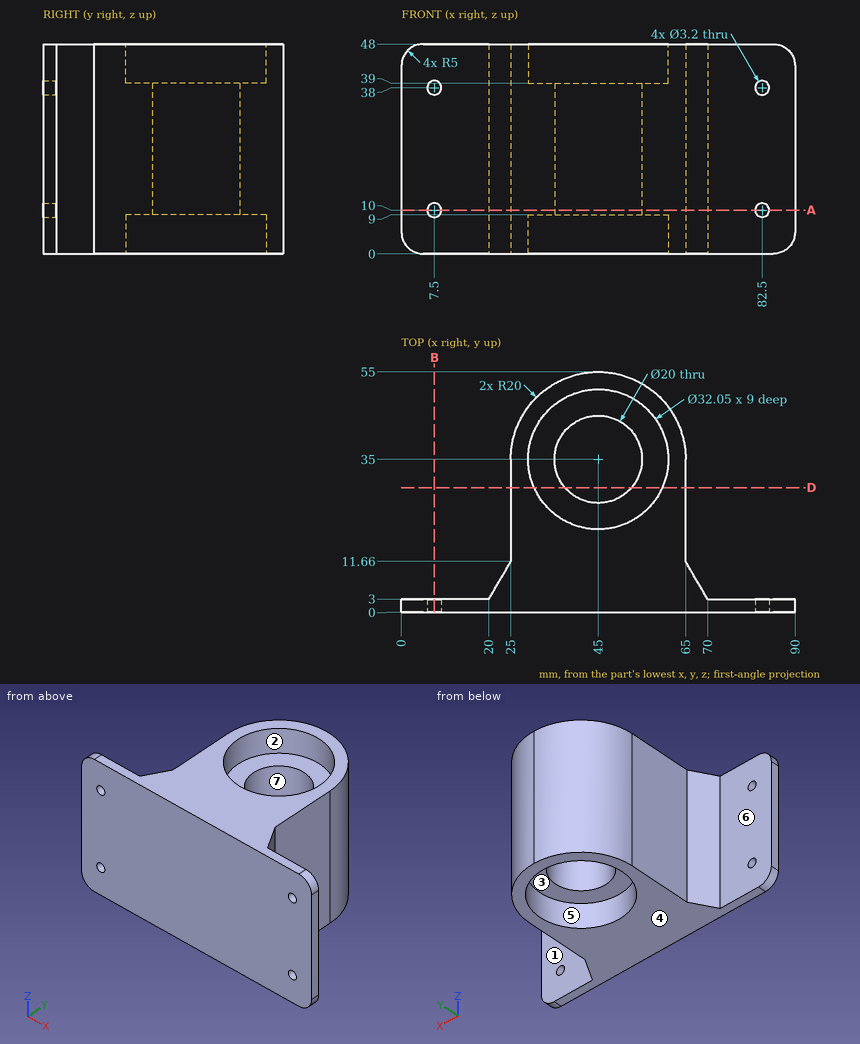
For this review, use the dimensioned drawing (mm, ordinates from the lowest corner) and the shaded views. A direction names the side the tool comes from. Give positions to 0.01 mm unless a question says otherwise; leave off trailing zeros. Write each loop counter-clockwise with the first axis right and the second up, starting at its lowest first coordinate (ties: lowest second). Pieces come first, ordered by that corner, then holes. Notation, with made-up numbers: M 55,27 L 69,27 A22 cw 69,48 Z; hole C -25,6.5 d10. An arc over 180 degrees is marked long. Answer as a JSON object with one key per item and string values. Group by question number.
Item 1: Consider section A-A on z = 10. Count the separate pieces of the cut face and the enclosed holes in it, plus the area to 3 significant figures.
Item 2: Consider section D-D on y = 28.5. Write out the cut boundary in (x, z), plus the area to 3 significant figures.
Item 3: Tool access review of the marked faces 1, 2 and 3: name each direction out of +Z, -Z, +X, -X, +Y, -Y from which nothing blocks a thin tool from reaching the whole face with its end or side.
Item 4: For probe 1 along X at (y, z) = (2.3, 38); probe 2 along Z at (x, y) = (82.5, 1.7); probe 3 along Y at (x, z) = (45, 24), list the stretches that pass through material, from the lowest coordinate up. Write a range as [from, to].
Item 5: For pin 1 Ø10 at (y, z) = (24, 21.5) entering from -X; pin 2 Ø1.9 at (x, z) = (7.5, 38) entering from +Y; pin 3 Ø6 at (y, z) = (7.5, 30.5) entering from +X; pin 4 Ø5 at (x, z) = (24.5, 42.5) entering from +Y, all flat-tipped, find the tip position at first contact; note any pin that passes through.
Item 6: Consider section B-B on x = 7.5. Write out the cut boundary in (y, z), plus the area to 3 significant figures.
Item 7: Draft analysis for pull direction Y (two halves, no side actions). For the marked faces 4, 5, 6 and 7, state which applies: +Y half, -Y half, draft (parallel to the pull), parting line (faces both ways), or undercut.
Check result:
{
 "1": {"separate pieces": "3", "enclosed holes": "1", "area": "1,890 mm^2"},
 "2": {"outline": "M 25,0 L 30.35,0 L 30.35,9 L 37.4,9 L 37.4,39 L 30.35,39 L 30.35,48 L 25,48 Z; M 52.6,9 L 59.65,9 L 59.65,0 L 65,0 L 65,48 L 59.65,48 L 59.65,39 L 52.6,39 Z", "area": "937 mm^2"},
 "3": {"face 1": "+Z, -Z, +X, +Y", "face 2": "+Z", "face 3": "-Z"},
 "4": {"probe 1": "x = [0, 5.9], [9.1, 80.9], [84.1, 90]", "probe 2": "z = [0, 8.4], [11.6, 36.4], [39.6, 48]", "probe 3": "y = [0, 25], [45, 55]"},
 "5": {"pin 1": "stops at x = 25", "pin 2": "passes through", "pin 3": "stops at x = 69.13", "pin 4": "stops at y = 43.72"},
 "6": {"outline": "M 0,0 L 3,0 L 3,8.4 L 0,8.4 Z; M 0,11.6 L 3,11.6 L 3,36.4 L 0,36.4 Z; M 0,39.6 L 3,39.6 L 3,48 L 0,48 Z", "area": "125 mm^2"},
 "7": {"face 4": "draft", "face 5": "undercut", "face 6": "+Y half", "face 7": "undercut"}
}
